Geometry check sheet. Reference: drawing and pictorial views, mm from the part's lowest x, y, z. Round coordinates to 2 decimals unless told otherwise and drop trailing zeros. Loops run counter-clockwise (first coordinate to the right, second up) from the corner with the lowest first, then second, coordinate; pieces in that order, holes last. Notation, with made-up numbers: M -8,69.5 L 26,69.5 A9 cw 26,83.5 Z; hole C -21.75,-33.5 d11. An arc over 180 degrees is marked long. One line per question, with ' | ' between items. Start each with the question number.
(1) Section check D-D (x = 20). Record the boundary of the cut face in (y, z), and give its area (3 significant figures).
(2) Draft check along Y on the marked faces 1 and 2. Enter one of: +Y half, -Y half, draft (parallel to the pull), parting line (faces both ways), or undercut.
(3) Section check B-B (y = 32.5). Record the boundary of the cut face in (x, z).
(4) Section check A-A (z = 3.5). Record the boundary of the cut face in (x, y), and give its area (3 significant figures).
(5) Thickness scan on probe 1 along Y at (x, z) = (128, 7.8); probe 2 along Y at (x, z) = (150, 7.8); probe 3 along Y at (x, z) = (162.5, 7.4). Record the ranges inside material, lowest first. Write a range as [from, to].
(6) Section check C-C (x = 137.5). Record the boundary of the cut face in (y, z), and give its area (3 significant figures).
(7) Go/stop test with flat-tipped pins: P1, Ø1.9, axis at x = 128, y = 36, coming from the +Z side; P2, Ø4, axis at x = 128, y = 4, coming from the -Z side. Record where each tip stops, or that it passes through.
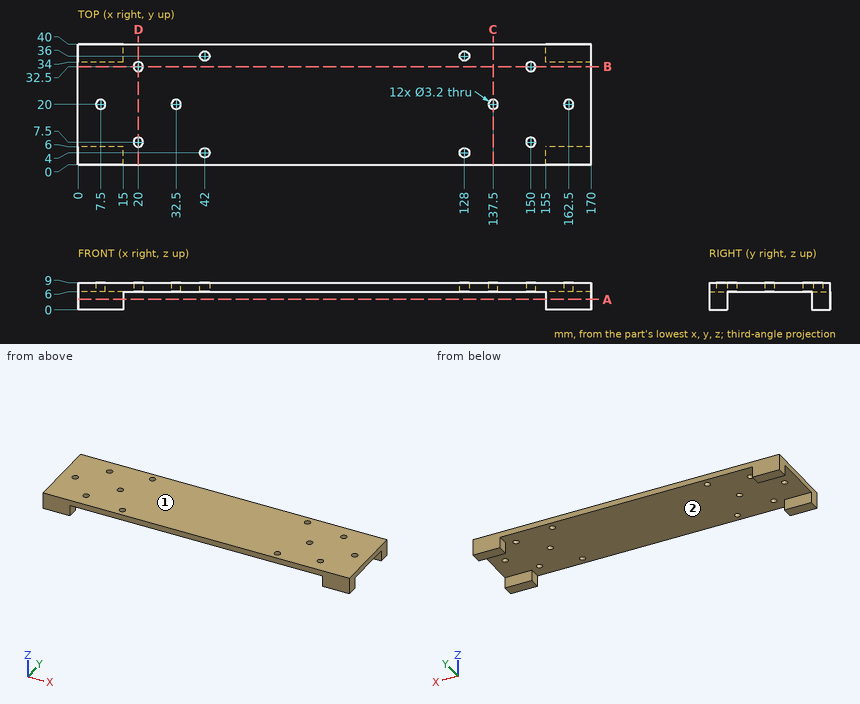
The answers:
1) outline: M 0,6 L 5.9,6 L 5.9,9 L 0,9 Z; M 9.1,6 L 30.9,6 L 30.9,9 L 9.1,9 Z; M 34.1,6 L 40,6 L 40,9 L 34.1,9 Z | area: 101 mm²
2) face 1: draft | face 2: undercut
3) outline: M 0,6 L 18.4,6 L 18.4,9 L 0,9 Z; M 21.6,6 L 148.4,6 L 148.4,9 L 21.6,9 Z; M 151.6,6 L 170,6 L 170,9 L 151.6,9 Z
4) outline: M 0,0 L 15,0 L 15,6 L 0,6 Z; M 0,34 L 15,34 L 15,40 L 0,40 Z; M 155,0 L 170,0 L 170,6 L 155,6 Z; M 155,34 L 170,34 L 170,40 L 155,40 Z | area: 360 mm²
5) probe 1: [0, 2.4], [5.6, 34.4], [37.6, 40] | probe 2: [0, 5.9], [9.1, 30.9], [34.1, 40] | probe 3: [0, 18.4], [21.6, 40]
6) outline: M 0,6 L 18.4,6 L 18.4,9 L 0,9 Z; M 21.6,6 L 40,6 L 40,9 L 21.6,9 Z | area: 110 mm²
7) P1: through | P2: z = 6
